Source: CAD feature listing. Evaluate the final solid. Frame: model axes, mm. A direction names the side the tool comes from. Give positions to 0.01 mm unless a question says otherwise; leave off trailing zeros. Write each loop counter-clockwise with the first axis right and the second up, starting at its lowest first coordinate (ties: lowest second). Pieces come first, ordered by that corner, then holes.
```python
from build123d import *

# Parameters (mm, degrees)
SKETCH010_R     = 10
PAD002_DEPTH    = 3
SKETCH011_R     = 8
POCKET008_DEPTH = 5
POCKET009_DEPTH = 1


with BuildPart() as part:
    # Sketch010 → Pad002 (new body)
    with BuildSketch(Plane.XY):
        Circle(SKETCH010_R)
    extrude(amount=PAD002_DEPTH)

    # Sketch011 → Pocket008 (cut)
    with BuildSketch(Plane.XY.offset(3)):
        Circle(SKETCH011_R)
    extrude(amount=-POCKET008_DEPTH, mode=Mode.SUBTRACT)

    # Sketch012 (on Face3 of Pocket008) → Pocket009 (cut)
    with BuildSketch(Plane.XY.offset(3)):
        with BuildLine():
            ThreePointArc((-7.07107, 7.071066), (-10, -2e-06), (-7.071068, -7.071068))
            Line((0, 0), (-7.071068, -7.071068))
            Line((-7.07107, 7.071066), (0, 0))
        make_face()
    extrude(amount=-POCKET009_DEPTH, mode=Mode.SUBTRACT)


with BuildPart() as part_1:
    # Body003 placement: moved
    add(part.part.moved(Location((-100, -75, 0))))


solid = part_1.part
```
1. Cut plane B-B, the plane y = -75. Return the cut outline in (x, z).
2. Cut plane A-A, the plane x = -100. Return the cut outline in (y, z), then the cut area to 3 significant figures.
3. Cut plane C-C, the plane z = 2.55. Return the cut outline in (x, y).
4. Line query: L1, parallel to X at y = -75, z = 1.05; L2, parallel to Y at x = -100, z = 0.9; L3, parallel to Z at x = -107, y = -81.25. Output: solid intervals per line, ascending.
5. Contact query for flat-ended pins moving along their axis: P1, Ø3.5, axis at x = -108, y = -72.5, coming from the +Z side; P2, Ø1.5, axis at y = -68.5, z = 1.5, coming from the -X side. Output: stop coordinate, or through.
6. Access query for faces 1 (the flat face through (-100, -66.8, 0)), 2 (the flat face through (-106.4, -68.6, 2.5)). Directions: +Z, -Z, +X, -X, +Y, -Y. A direction counts if a zero-diameter tool reaches every point of the face in a straight line with its end or side. Return the directions, or none.
7. Cut plane D-D, the plane y = -68.5. Return the cut outline in (x, z), then the cut area to 3 significant figures.
8. Mould query, pull axis Y, two halves, no side actions, for faces 3 (the cylindrical face through (-90.763, -78.83, 1.479)), 4 (the flat face through (-92, -77, 3)), 5 (the flat face through (-108.3, -74.9, 2)). Classes: +Y half, -Y half, draft (parallel to the pull), parting line (faces both ways), or undercut.
Response values:
1. outline: (-110, 0) - (-108, 0) - (-108, 2) - (-110, 2) - close; (-92, 0) - (-90, 0) - (-90, 3) - (-92, 3) - close
2. outline: (-85, 0) - (-83, 0) - (-83, 3) - (-85, 3) - close; (-67, 0) - (-65, 0) - (-65, 3) - (-67, 3) - close
2. area: 12.0 mm2
3. outline: (-107.07, -82.07) arc R10 ccw (long way) to (-107.07, -67.93) - (-105.66, -69.34) arc R8 cw (long way) to (-105.66, -80.66) - close
4. L1: x = -110 to -108, -92 to -90
4. L2: y = -85 to -83, -67 to -65
4. L3: z = 0 to 2
5. P1: stops at z = 2
5. P2: stops at x = -108.18
6. face 1: -Z, +X, -X, +Y, -Y
6. face 2: +Z, -X
7. outline: (-107.6, 0) - (-104.66, 0) - (-104.66, 3) - (-106.5, 3) - (-106.5, 2) - (-107.6, 2) - close; (-95.34, 0) - (-92.4, 0) - (-92.4, 3) - (-95.34, 3) - close
7. area: 16.5 mm2
8. face 3: parting line
8. face 4: draft
8. face 5: undercut
